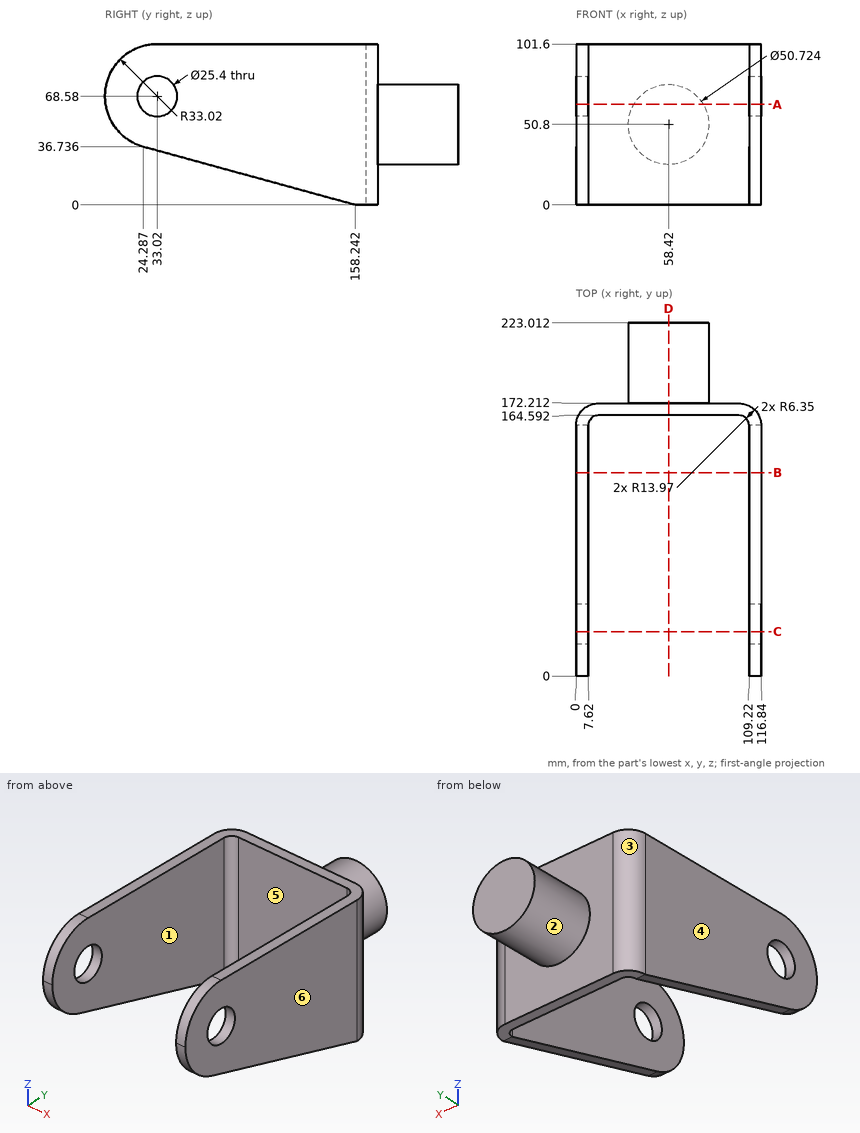
Geometry: see drawing. Coordinates: mm, zero at the bounding-box minimum. A direction names the side the tool comes from. Round coordinates to 2 decimals unless told otherwise and drop trailing zeros. Order: outer loops, then holes, each group sorted by start corner. A loop starts at its lowest first (then second) coordinate and runs counter-clockwise, first axis right, second up. Notation, with made-up numbers: (46.5, -30.5) - (79.5, -30.5) arc R10 ccw to (79.5, -16.5) - close; hole circle Ø1 at (82, 0.25). An arc over 180 degrees is marked (long way). Use a Markdown table: item, result. Add a question column.
1. Section query C-C (y = 28). Return the cut outline in (x, z).
2. Line query: probe 1 along X at (y, z) = (80, 56.5); probe 2 along Y at (x, z) = (112, 68) (1 decimal); probe 3 along Y at (x, z) = (5, 68.58). Output: solid intervals per line, ascending.
3. Set-up query: the marked faces 1, 2 and 3. Return all of +Z, -Z, +X, -X, +Y, -Y with unobstructed straight access to the full face (end or side cutting, diameter ignored); none if empty.
4. Mould query, pull axis X, two halves, no side actions, for the marked faces 4, 5 and 6. Classes: +X half, -X half, draft (parallel to the pull), parting line (faces both ways), or undercut.
5. First-contact query: pin 1 (6 mm diameter, centred on x = 89.5, z = 68, fed in from -Y); pin 2 (1 mm diameter, centred on x = 65, z = 85, fed in from +Y); pin 3 (15 mm diameter, centred on y = 33.02, z = 68.58, fed in from +X); pin 4 (1.5 mm diameter, centred on y = 192, z = 30, fed in from +X). Flat tips, straight axial feed; report the tip coordinate or a pass-through.
6. Section query D-D (x = 58.42). Return the cut outline in (y, z), then the cut area to 3 significant figures.
7. Section query B-B (y = 128.5). Return the cut outline in (x, z).
8. Section query A-A (z = 63.5). Return the cut outline in (x, y).
Derived:
| question | item | result |
|---|---|---|
| 1 | outline | (0, 35.72) - (7.62, 35.72) - (7.62, 56.91) - (0, 56.91) - close; (0, 80.25) - (7.62, 80.25) - (7.62, 101.22) - (0, 101.22) - close; (109.22, 35.72) - (116.84, 35.72) - (116.84, 56.91) - (109.22, 56.91) - close; (109.22, 80.25) - (116.84, 80.25) - (116.84, 101.22) - (109.22, 101.22) - close |
| 2 | probe 1 | 0 to 7.62, 109.22 to 116.84 |
| 2 | probe 2 | 0 to 20.3, 45.7 to 168.8 |
| 2 | probe 3 | 0 to 20.32, 45.72 to 168.95 |
| 3 | face 1 | +Z, -Z, -Y |
| 3 | face 2 | +Y |
| 3 | face 3 | +Z, -Z, -X, +Y |
| 4 | face 4 | -X half |
| 4 | face 5 | undercut |
| 4 | face 6 | +X half |
| 5 | pin 1 | y = 164.59 |
| 5 | pin 2 | y = 172.21 |
| 5 | pin 3 | through |
| 5 | pin 4 | x = 73.95 |
| 6 | outline | (164.59, 0) - (172.21, 0) - (172.21, 25.44) - (223.01, 25.44) - (223.01, 76.16) - (172.21, 76.16) - (172.21, 101.6) - (164.59, 101.6) - close |
| 6 | area | 3,350 mm2 |
| 7 | outline | (0, 8.16) - (7.62, 8.16) - (7.62, 101.6) - (0, 101.6) - close; (109.22, 8.16) - (116.84, 8.16) - (116.84, 101.6) - (109.22, 101.6) - close |
| 8 | outline | (0, 0.39) - (7.62, 0.39) - (7.62, 21.38) - (0, 21.38) - close; (0, 44.66) - (7.62, 44.66) - (7.62, 158.24) arc R6.35 cw to (13.97, 164.59) - (102.87, 164.59) arc R6.35 cw to (109.22, 158.24) - (109.22, 44.66) - (116.84, 44.66) - (116.84, 158.24) arc R13.97 ccw to (102.87, 172.21) - (80.37, 172.21) - (80.37, 223.01) - (36.47, 223.01) - (36.47, 172.21) - (13.97, 172.21) arc R13.97 ccw to (0, 158.24) - close; (109.22, 0.39) - (116.84, 0.39) - (116.84, 21.38) - (109.22, 21.38) - close |
